Can you work these out from the model? Positions are in its coordinate system, mm. Face numbers are marked on the shaded views. A direction names the side the tool comes from. Give positions to 0.01 mm unless a question says otherwise; leave off trailing zeros. Order: outer loops, then holes, each group sorted by start corner. A loop starts at its lowest first (then second) coordinate and runs counter-clockwise, first axis right, second up. Notation, with made-up numbers: (35.5, 47.25) - (62.5, 47.25) arc R22 ccw to (62.5, 70.25) - close; hole circle Ø9 at (-9.75, 33). An arc over 180 degrees is marked (long way). Return JSON: item names as keys, results as strings.
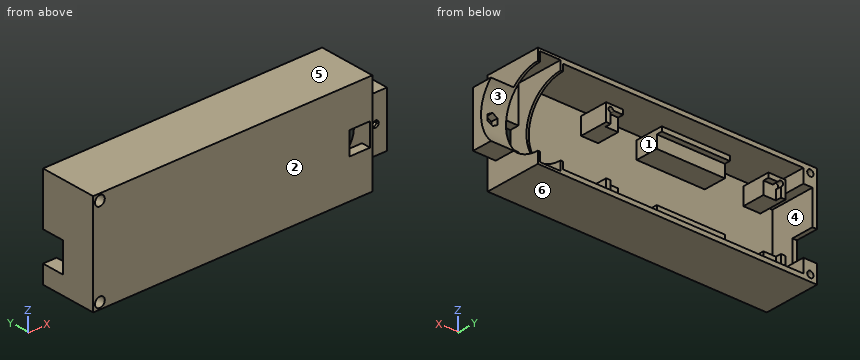
```python
from build123d import *

# Parameters (mm, degrees)
SKETCH3_W           = 520.7
SKETCH3_H           = 111.76
BOSS_EXTRUDE1_DEPTH = 63.5
CUT_EXTRUDE1_START  = 6.35
SKETCH2_W           = 77.47
SKETCH2_H           = 77.47
CUT_EXTRUDE1_DEPTH  = 111.76
SKETCH4_R           = 50.8
CUT_EXTRUDE2_DEPTH  = 156.718
SKETCH5_R           = 43.18
CUT_EXTRUDE3_DEPTH  = 355.6
SKETCH6_W           = 279.4
SKETCH6_H           = 101.6
CUT_EXTRUDE4_DEPTH  = 50.8
CUT_EXTRUDE5_DEPTH  = 174.244
SKETCH9_W           = 25.4
SKETCH9_H           = 60.96
CUT_EXTRUDE6_DEPTH  = 10.16
BOSS_EXTRUDE2_REACH = 310.043
SKETCH11_W          = 15.24
SKETCH11_H          = 20.32
SKETCH10_R          = 3.5
CUT_EXTRUDE7_DEPTH  = 76.2
SKETCH10_3_R        = 5.5
CUT_EXTRUDE8_DEPTH  = 45.72
SKETCH13_R          = 3.5
CUT_EXTRUDE9_DEPTH  = 34.448
CUT_EXTRUDE10_START = -2.54
SKETCH13_3_R        = 3.5
CUT_EXTRUDE10_DEPTH = 34.448
SKETCH14_W          = 13.97
SKETCH14_H          = 13.97
SKETCH14_W_2        = 19.05
SKETCH14_H_2        = 19.05
SKETCH14_W_3        = 76.2
BOSS_EXTRUDE3_DEPTH = 25.4
SKETCH14_3_W        = 76.2
SKETCH14_3_H        = 5.08
BOSS_EXTRUDE4_DEPTH = 31.75
SKETCH16_W          = 22.86
SKETCH16_H          = 106.68
CUT_EXTRUDE12_DEPTH = 53.34
SKETCH17_W          = 22.86
SKETCH17_H          = 25.4
CUT_EXTRUDE13_DEPTH = 52.54
SKETCH18_W          = 33.02
SKETCH18_H          = 25.4
CUT_EXTRUDE14_DEPTH = 17.018
SKETCH19_R          = 2.54
CUT_EXTRUDE15_DEPTH = 23.876
FILLET1_R           = 2.54


with BuildPart() as part:
    # Sketch3 → Boss-Extrude1 (new body)
    with BuildSketch(Plane(origin=(0, 0, 0), x_dir=(1, 0, 0), z_dir=(0, 1, 0))):
        with Locations((209.55, 36.195)):
            Rectangle(SKETCH3_W, SKETCH3_H)
    extrude(amount=BOSS_EXTRUDE1_DEPTH)

    # Sketch2 → Cut-Extrude1 (cut)
    with BuildSketch(Plane(origin=(0, 0, 0), x_dir=(1, 0, 0), z_dir=(0, 1, 0)).offset(CUT_EXTRUDE1_START)):
        with Locations((412.75, 36.195)):
            Rectangle(SKETCH2_W, SKETCH2_H)
    extrude(amount=CUT_EXTRUDE1_DEPTH, mode=Mode.SUBTRACT)

    # Sketch4 → Cut-Extrude2 (cut)
    with BuildSketch(Plane.XY.offset(19.685)):
        with Locations((330.2, 63.5)):
            Circle(SKETCH4_R)
        Polygon((469.9, 12.7), (330.2, 12.7), (279.4, 63.5), (469.9, 63.5), align=None)
    extrude(amount=-CUT_EXTRUDE2_DEPTH, mode=Mode.SUBTRACT)

    # Sketch5 → Cut-Extrude3 (cut)
    with BuildSketch(Plane(origin=(0, 0, 0), x_dir=(0, 0, -1), z_dir=(1, 0, 0))):
        with Locations((36.195, 63.5)):
            Circle(SKETCH5_R)
    extrude(amount=CUT_EXTRUDE3_DEPTH, mode=Mode.SUBTRACT)

    # Sketch6 → Cut-Extrude4 (cut)
    with BuildSketch(Plane(origin=(0, 63.5, 0), x_dir=(1, 0, 0), z_dir=(0, 1, 0))):
        with Locations((93.98, 36.195)):
            Rectangle(SKETCH6_W, SKETCH6_H)
    extrude(amount=-CUT_EXTRUDE4_DEPTH, mode=Mode.SUBTRACT)

    # Sketch7 → Cut-Revolve1 (revolve, cut)
    with BuildSketch(Plane(origin=(0, 63.5, 0), x_dir=(1, 0, 0), z_dir=(0, 1, 0))):
        with BuildLine():
            Line((241.3, -13.805), (245.161436971, -13.805))
            ThreePointArc((245.161436971, -13.805), (245.979341863, -10.401680901), (246.739500346, -6.985))
            Line((246.739500346, -6.985), (241.3, -6.985))
            Line((241.3, -6.985), (241.3, -13.805))
        make_face()
    revolve(axis=Axis((-45.72, 63.5, -36.195), (1, 0, 0)), mode=Mode.SUBTRACT)

    # Sketch8 → Cut-Extrude5 (cut)
    with BuildSketch(Plane.XZ):
        Polygon((261.62, 19.685), (261.62, -5.715), (287.02, -5.715), (287.02, -66.675), (261.62, -66.675), (261.62, -92.075), (609.54801076, -173.862508288), (609.54801076, 88.425228921), align=None)
    extrude(amount=-CUT_EXTRUDE5_DEPTH, mode=Mode.SUBTRACT)

    # Sketch9 → Cut-Extrude6 (cut)
    with BuildSketch(Plane.XZ):
        with Locations((274.32, -36.195)):
            Rectangle(SKETCH9_W, SKETCH9_H)
    extrude(amount=-CUT_EXTRUDE6_DEPTH, mode=Mode.SUBTRACT)

    # Sketch11 → Boss-Extrude2 (add, up to next)
    with BuildSketch(Plane(origin=(0, 63.5, 0), x_dir=(1, 0, 0), z_dir=(0, 1, 0)), mode=Mode.PRIVATE) as boss_extrude2_sk1:
        with Locations((-43.18, 81.915)):
            Rectangle(SKETCH11_W, SKETCH11_H)
    boss_extrude2_tool1 = extrude(boss_extrude2_sk1.sketch, amount=-BOSS_EXTRUDE2_REACH, mode=Mode.PRIVATE) - part.part
    # Sketch11 → Boss-Extrude2 (add, up to next)
    with BuildSketch(Plane(origin=(0, 63.5, 0), x_dir=(1, 0, 0), z_dir=(0, 1, 0)), mode=Mode.PRIVATE) as boss_extrude2_sk2:
        with Locations((-43.18, -9.525)):
            Rectangle(SKETCH11_W, SKETCH11_H)
    boss_extrude2_tool2 = extrude(boss_extrude2_sk2.sketch, amount=-BOSS_EXTRUDE2_REACH, mode=Mode.PRIVATE) - part.part
    add(boss_extrude2_tool1.solids().sort_by_distance((-43.18, 63.5, -81.915))[0])
    add(boss_extrude2_tool2.solids().sort_by_distance((-43.18, 63.5, 9.525))[0])

    # Sketch10 → Cut-Extrude7 (cut)
    with BuildSketch(Plane.XZ):
        with Locations(Location((-43.346, -84.963, 0), (0, 0, 270))):
            Circle(SKETCH10_R)
        with Locations(Location((-43.346, 12.573, 0), (0, 0, 270))):
            Circle(SKETCH10_R)
    extrude(amount=-CUT_EXTRUDE7_DEPTH, mode=Mode.SUBTRACT)

    # Sketch10_3 → Cut-Extrude8 (cut)
    with BuildSketch(Plane.XZ):
        with Locations(Location((-43.346, 12.573, 0), (0, 0, 270))):
            Circle(SKETCH10_3_R)
        with Locations(Location((-43.346, -84.963, 0), (0, 0, 270))):
            Circle(SKETCH10_3_R)
    extrude(amount=-CUT_EXTRUDE8_DEPTH, mode=Mode.SUBTRACT)

    # Sketch13 → Cut-Extrude9 (cut)
    with BuildSketch(Plane.XZ.offset(-10.16)):
        with Locations(Location((274.32, -36.195, 0), (0, 0, 270))):
            Circle(SKETCH13_R)
    extrude(amount=-CUT_EXTRUDE9_DEPTH, mode=Mode.SUBTRACT)

    # Sketch13_3 → Cut-Extrude10 (cut)
    with BuildSketch(Plane.XZ.offset(-10.16).offset(CUT_EXTRUDE10_START)):
        Polygon((268.82, -39.370426481), (274.32, -42.545852961), (279.82, -39.370426481), (279.82, -33.019573519), (274.32, -29.844147039), (268.82, -33.019573519), align=None)
        with Locations(Location((274.32, -36.195, 0), (0, 0, 270))):
            Circle(SKETCH13_3_R, mode=Mode.SUBTRACT)
    extrude(amount=-CUT_EXTRUDE10_DEPTH, mode=Mode.SUBTRACT)

    # Sketch14 → Boss-Extrude3 (add)
    with BuildSketch(Plane(origin=(0, 12.7, 0), x_dir=(1, 0, 0), z_dir=(0, 1, 0))):
        Polygon((149.25, 82.275), (149.25, 77.195), (163.22, 77.195), (163.22, 63.225), (168.3, 63.225), (168.3, 82.275), align=None)
        with Locations((156.235, 70.21)):
            Rectangle(SKETCH14_W, SKETCH14_H)
        with Locations((-22.835, 72.75)):
            Rectangle(SKETCH14_W_2, SKETCH14_H_2)
        with Locations((158.775, -0.36)):
            Rectangle(SKETCH14_W_2, SKETCH14_H_2)
        with Locations((-22.835, -0.36)):
            Rectangle(SKETCH14_W_2, SKETCH14_H_2)
        with Locations((67.97, 72.75)):
            Rectangle(SKETCH14_W_3, SKETCH14_H_2)
        with Locations((67.97, -0.36)):
            Rectangle(SKETCH14_W_3, SKETCH14_H_2)
    extrude(amount=BOSS_EXTRUDE3_DEPTH)

    # Sketch14_3 → Boss-Extrude4 (add)
    with BuildSketch(Plane(origin=(0, 12.7, 0), x_dir=(1, 0, 0), z_dir=(0, 1, 0))):
        Polygon((-13.31, -4.805), (-27.28, -4.805), (-27.28, 9.165), (-32.36, 9.165), (-32.36, -9.885), (-13.31, -9.885), align=None)
        with Locations((67.97, -7.345)):
            Rectangle(SKETCH14_3_W, SKETCH14_3_H)
        Polygon((-32.36, 63.225), (-27.28, 63.225), (-27.28, 77.195), (-13.31, 77.195), (-13.31, 82.275), (-32.36, 82.275), align=None)
        Polygon((163.22, -4.805), (149.25, -4.805), (149.25, -9.885), (168.3, -9.885), (168.3, 9.165), (163.22, 9.165), align=None)
        with Locations((67.97, 79.735)):
            Rectangle(SKETCH14_3_W, SKETCH14_3_H)
        Polygon((149.25, 82.275), (149.25, 77.195), (163.22, 77.195), (163.22, 63.225), (168.3, 63.225), (168.3, 82.275), align=None)
    extrude(amount=BOSS_EXTRUDE4_DEPTH)

    # Sketch16 → Cut-Extrude12 (cut)
    with BuildSketch(Plane(origin=(0, 63.5, 0), x_dir=(1, 0, 0), z_dir=(0, 1, 0))):
        with Locations((247.65, 36.195)):
            Rectangle(SKETCH16_W, SKETCH16_H)
    extrude(amount=-CUT_EXTRUDE12_DEPTH, mode=Mode.SUBTRACT)

    # Sketch17 → Cut-Extrude13 (cut)
    with BuildSketch(Plane(origin=(0, 10.16, 0), x_dir=(1, 0, 0), z_dir=(0, 1, 0))):
        with Locations((247.65, 36.195)):
            Rectangle(SKETCH17_W, SKETCH17_H)
    extrude(amount=-CUT_EXTRUDE13_DEPTH, mode=Mode.SUBTRACT)

    # Sketch18 → Cut-Extrude14 (cut)
    with BuildSketch(Plane.ZY.offset(50.8)):
        with Locations((-55.245, 50.8)):
            Rectangle(SKETCH18_W, SKETCH18_H)
    extrude(amount=-CUT_EXTRUDE14_DEPTH, mode=Mode.SUBTRACT)

    # Sketch19 → Cut-Extrude15 (cut)
    with BuildSketch(Plane(origin=(0, 38.1, 0), x_dir=(1, 0, 0), z_dir=(0, 1, 0))):
        with Locations((-27.28, 77.195)):
            Circle(SKETCH19_R)
        with Locations((163.22, 77.195)):
            Circle(SKETCH19_R)
        with Locations((163.22, -4.805)):
            Circle(SKETCH19_R)
        with Locations((-27.28, -4.805)):
            Circle(SKETCH19_R)
    extrude(amount=CUT_EXTRUDE15_DEPTH, mode=Mode.SUBTRACT)

    # Fillet1
    fillet1_edges = [part.edges().sort_by_distance(p)[0] for p in [
        (-27.28, 41.275, 2.265),
        (-24.74, 41.275, 4.805),
        (163.22, 41.275, 2.265),
        (160.68, 41.275, 4.805),
        (163.22, 41.275, -74.655),
        (160.68, 41.275, -77.195),
        (-27.28, 41.275, -74.655),
        (-24.74, 41.275, -77.195),
    ]]
    fillet(fillet1_edges, radius=FILLET1_R)


solid = part.part
```
1. On a 3-axis mill with a long thin cutter (end or side, diameter ignored), from which of +Z, -Z, +X, -X, +Y, -Y can I reach the whole of each face in a straight line? I mean the marked faces 1, 2 and 3. Say none if no direction works.
Checks:
{"face 1": "+Y", "face 2": "+Z, -Z, +X, -X, -Y", "face 3": "+X, +Y"}
2. Suppose I cut it at A-A (y = 51). List the corners of the cut face in (x, z) for me (3 decimals).
Checks:
{"outline": "(-50.8, -92.075) - (261.62, -92.075) - (261.62, -77.526) - (259.08, -77.526) - (259.08, -89.535) - (236.22, -89.535) - (236.22, -77.526) - (233.68, -77.526) - (233.68, -86.995) - (-35.56, -86.995) - (-35.56, -71.755) - (-50.8, -71.755) - close; (-50.8, -38.735) - (-45.72, -38.735) - (-45.72, -0.635) - (-35.56, -0.635) - (-35.56, 14.605) - (233.68, 14.605) - (233.68, 5.136) - (236.22, 5.136) - (236.22, 17.145) - (259.08, 17.145) - (259.08, 5.136) - (261.62, 5.136) - (261.62, 19.685) - (-50.8, 19.685) - close; hole circle Ø7 at (-43.346, -84.963); hole circle Ø7 at (-43.346, 12.573)"}
3. Thinking about a two-plate mould opening in Z: for the marked faces 4, 5 and 6, which applies, +Z half, -Z half, draft (parallel to the pull), parting line (faces both ways), or undercut?
Checks:
{"face 4": "undercut", "face 5": "+Z half", "face 6": "-Z half"}
4. For pin 1 Ø1 at (y, z) = (15.5, -80.5) entering from +X; pin 2 Ø20.5 at (x, z) = (277, -36.5) entering from -Y; pin 3 Ø8 at (y, z) = (52.5, -73.5) entering from +X, each with a flat end and sliding along its axis, tell me the tip position at first contact or that it passes through.
Checks:
{"pin 1": "x = 261.62", "pin 2": "y = 10.16", "pin 3": "x = -35.56"}
5. If I drill on L1, parallel to X at y = 21.5, z = -46.5; L2, parallel to Z at x = 59.5, y = 18 (3 decimals); L3, parallel to X at y = 22, z = -2, over which ranges is the centre line in solid material (lowest first)? Write a range as [from, to].
Checks:
{"L1": "[-50.8, -45.72], [233.68, 236.22], [259.08, 287.02]", "L2": "[-92.075, -86.995], [-82.275, -63.225], [-9.165, 9.885], [14.605, 19.685]", "L3": "[-50.8, -45.72], [-32.36, -13.31], [29.87, 106.07], [149.25, 168.3], [233.68, 236.22], [259.08, 261.62]"}
6. Suppose I cut it at C-C (z = -17). List the corners of the cut face in (x, y) for me, plus the area to 3 significant figures.
Checks:
{"outline": "(-50.8, 0) - (261.62, 0) - (261.62, 10.16) - (287.02, 10.16) - (287.02, 24.82) - (259.08, 24.82) - (259.08, 10.16) - (236.22, 10.16) - (236.22, 24.82) - (233.68, 24.82) - (233.68, 12.7) - (-45.72, 12.7) - (-45.72, 63.5) - (-50.8, 63.5) - close", "area": "4,600 mm^2"}
7. Suppose I cut it at D-D (y = 26). State how many separate pieces and enclosed holes the cut face has, plus the area to 3 significant figures.
Checks:
{"separate pieces": "7", "enclosed holes": "2", "area": "8,810 mm^2"}
8. Suppose I cut it at B-B (x = -7.5). List the corners of the cut face in (y, z) for me (3 decimals).
Checks:
{"outline": "(0, -92.075) - (63.5, -92.075) - (63.5, -86.995) - (12.7, -86.995) - (12.7, 14.605) - (63.5, 14.605) - (63.5, 19.685) - (0, 19.685) - close"}
